Answer from the drawing. Dimensions are ordinates in mm from the lowest x, y and z of the part. Give positions to 0.01 mm unless a question says otherwise; leave off trailing zeros. Write each loop counter-clockwise with the first axis right and the second up, starting at its lowest first coordinate (ties: lowest second). Pieces come first, ordered by that corner, then holes. Notation, with made-up numbers: M 76,9.25 L 115,9.25 A26 ccw 115,48.25 Z; hole C -26,10 d6. An arc over 180 degrees is marked long. Put each result on its own line as item: value.
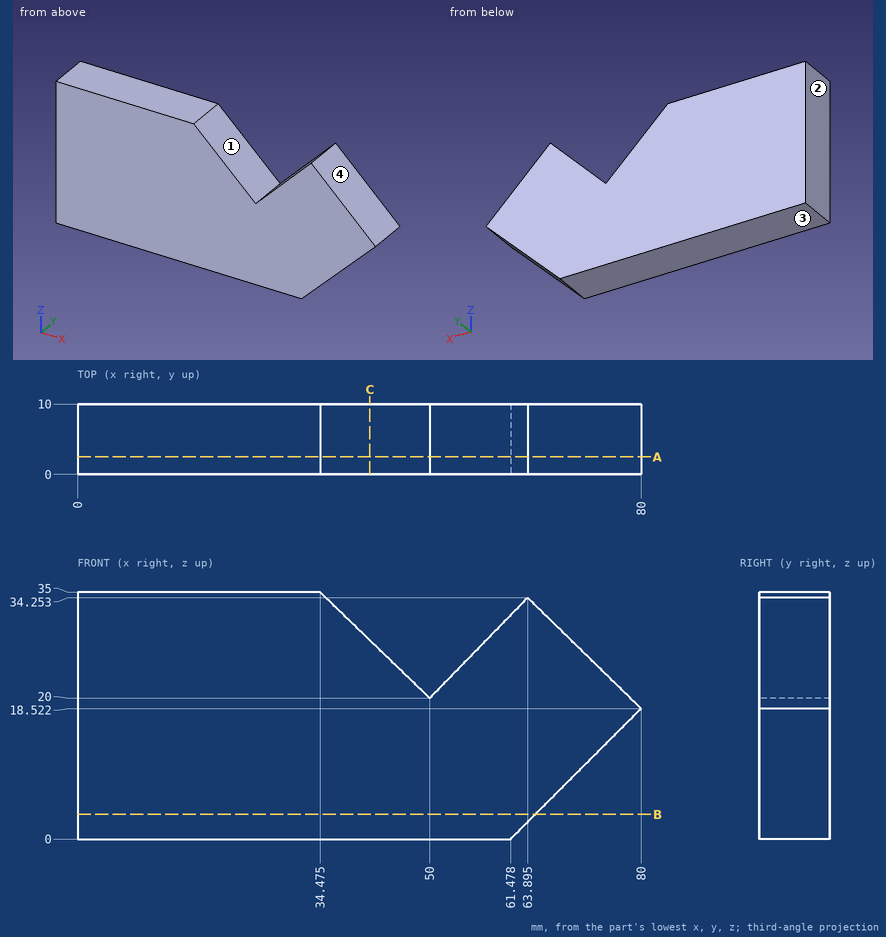
(1) For a pull along X with two mould halves and no side action, classify the marked faces 1, 2, 3 and 4 as +X half, -X half, draft (parallel to the pull), parting line (faces both ways), or undercut.
Result:
face 1: undercut
face 2: -X half
face 3: draft
face 4: +X half
(2) Given pin 1 Ø1 at (x, y) = (47.5, 5.5) entering from +Z; pin 2 Ø6 at (x, y) = (39.5, 2) entering from +Z, each flat-ended and moving along its own axis, determine where each tip first touches the part or whether it passes through.
Result:
pin 1: stops at z = 22.9
pin 2: stops at z = 33.04
(3) Section A-A on y = 2.5 is taken. Determine the outline of the cut face in (x, z) (1 decimal), and give its area (3 significant figures).
Result:
outline: M 0,0 L 61.5,0 L 80,18.5 L 63.9,34.3 L 50,20 L 34.5,35 L 0,35 Z
area: 2,260 mm²
(4) Section B-B on z = 3.5 is taken. Determine the outline of the cut face in (x, y).
Result:
outline: M 0,0 L 64.98,0 L 64.98,10 L 0,10 Z
(5) Section C-C on x = 41.5 is taken. Determine the outline of the cut face in (y, z).
Result:
outline: M 0,0 L 10,0 L 10,28.21 L 0,28.21 Z
(6) Straight lines are drawn through the part: line 1 along X through (y, z) = (2.5, 23) (1 decimal); line 2 along X through (y, z) = (6.75, 20.5) (1 decimal); line 3 along Z through (x, y) = (51.5, 2). For each, find the intervals that lie inside material, in ascending order. Write a range as from..to.
Result:
line 1: x = 0..46.9, 52.9..75.4
line 2: x = 0..49.5, 50.5..78
line 3: z = 0..21.54
